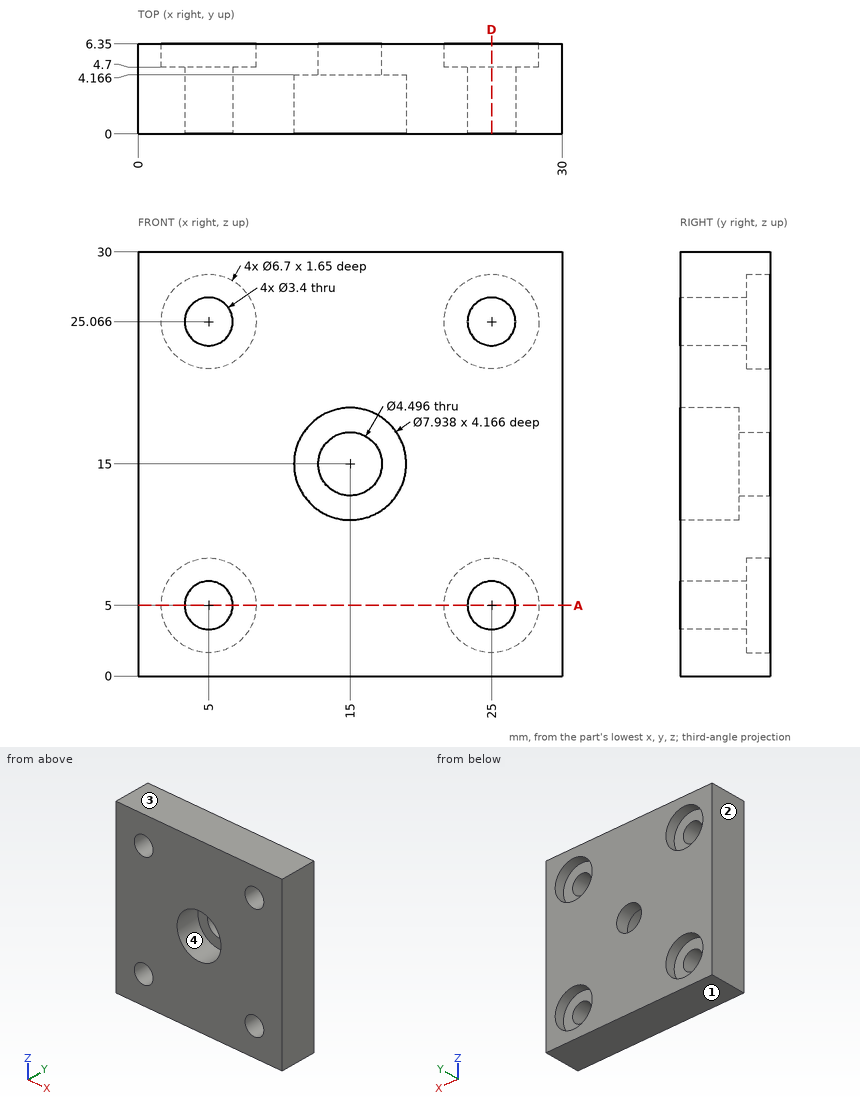
Print and shaded views of the part. All mm, measured from the part's lowest x, y and z. Coordinates: 2 decimals unless noted, no trailing zeros. Write each loop counter-clockwise with the first axis right and the second up, starting at its lowest first coordinate (ties: lowest second). Pieces come first, ordered by that corner, then holes. Notation, with made-up numbers: M 78,26.25 L 107,26.25 A31 ccw 107,57.25 Z; hole C 80,15.5 d7. An arc over 180 degrees is marked long. Return JSON: item names as keys, results as strings.
1. Saw through at A-A, the plane z = 5. Write the cut outline in (x, y).
Determined:
{"outline": "M 0,0 L 3.3,0 L 3.3,4.7 L 1.65,4.7 L 1.65,6.35 L 0,6.35 Z; M 6.7,0 L 23.3,0 L 23.3,4.7 L 21.65,4.7 L 21.65,6.35 L 8.35,6.35 L 8.35,4.7 L 6.7,4.7 Z; M 26.7,0 L 30,0 L 30,6.35 L 28.35,6.35 L 28.35,4.7 L 26.7,4.7 Z"}
2. Saw through at D-D, the plane x = 25. Count the separate pieces of the cut face and the enclosed holes in it.
Determined:
{"separate pieces": "3", "enclosed holes": "0"}
3. Probe L1, parallel to X at y = 2.5, z = 5; L2, parallel to Z at x = 5, y = 2.3 (1 decimal); L3, parallel to Z at x = 24, y = 4.25 (1 decimal). List the from-to ranges inside material, lowest first.
Determined:
{"L1": "0 to 3.3, 6.7 to 23.3, 26.7 to 30", "L2": "0 to 3.3, 6.7 to 23.4, 26.8 to 30", "L3": "0 to 3.6, 6.4 to 23.7, 26.4 to 30"}
4. Pull direction Z, two halves, no side cores. Call the marked faces 1, 2, 3 and 4: pulls with the +Z half, pulls with the -Z half, needs draft (parallel to the pull), parting line crosses it, or undercut.
Determined:
{"face 1": "pulls with the -Z half", "face 2": "needs draft", "face 3": "pulls with the +Z half", "face 4": "undercut"}
5. Flat gauge pins, fed straight in: pin 1 Ø5.5 at (x, z) = (24.5, 5) entering from +Y; pin 2 Ø7 at (x, z) = (15, 15) entering from -Y. Where does each tip first touch, or does it go through?
Determined:
{"pin 1": "y = 4.7", "pin 2": "y = 4.17"}
